Geometry: final body of the model. Coordinates: model frame, mm. A direction names the side the tool comes from. Coordinates: 2 decimals unless noted, no trailing zeros. Order: outer loops, then holes, each group sorted by start corner. A loop starts at its lowest first (then second) coordinate and runs counter-clockwise, first axis right, second up. Notation, with made-up numbers: (70.25, 65) -> (109.25, 65) arc R19 cw to (109.25, 89) -> close; hole circle Ø8 at (14.5, 6). An arc over 180 degrees is marked (long way). Use one line per item in the form item = value.
```python
from build123d import *

# Parameters (mm, degrees)
BOSS_EXTRUDE1_DEPTH = 14.5
CUT_EXTRUDE1_DEPTH  = 4
CUT_EXTRUDE2_DEPTH  = 4


with BuildPart() as part:
    # Sketch1 → Boss-Extrude1 (new body)
    with BuildSketch(Plane(origin=(0, 0, 0), x_dir=(0, 0, -1), z_dir=(1, 0, 0))):
        Polygon((0, 20), (0, 0), (20, 0), (20, 3), (3, 3), (3, 20), align=None)
    extrude(amount=-BOSS_EXTRUDE1_DEPTH)

    # Sketch2 → Cut-Extrude1 (cut, through all)
    with BuildSketch(Plane(origin=(0, 0, -3), x_dir=(-1, 0, 0), z_dir=(0, 0, -1))):
        with BuildLine():
            Line((5.5, 12.75), (9, 12.75))
            ThreePointArc((9, 12.75), (11.75, 10), (9, 7.25))
            Line((9, 7.25), (5.5, 7.25))
            ThreePointArc((5.5, 7.25), (2.75, 10), (5.5, 12.75))
        make_face()
    extrude(amount=-CUT_EXTRUDE1_DEPTH, mode=Mode.SUBTRACT)

    # Sketch3 → Cut-Extrude2 (cut, through all)
    with BuildSketch(Plane(origin=(0, 3, 0), x_dir=(1, 0, 0), z_dir=(0, 1, 0))):
        with BuildLine():
            Line((-5.5, 12.25), (-9, 12.25))
            ThreePointArc((-9, 12.25), (-11.75, 15), (-9, 17.75))
            Line((-9, 17.75), (-5.5, 17.75))
            ThreePointArc((-5.5, 17.75), (-2.75, 15), (-5.5, 12.25))
        make_face()
    extrude(amount=-CUT_EXTRUDE2_DEPTH, mode=Mode.SUBTRACT)


solid = part.part
```
1) Material intervals for probe 1 along Z at (x, y) = (-8.25, 14.75); probe 2 along Y at (x, z) = (-5.25, -4); probe 3 along Y at (x, z) = (-11, -2), sorted ascending. Write a range as from..to.
Results found:
probe_1 = -3..0
probe_2 = 0..3
probe_3 = 0..8.11, 11.89..20
2) Access query for faces 1 (the flat face through (-7, 3, -12)), 2 (the flat face through (-7, 7.25, -2)), 3 (the cylindrical face through (-11.75, 1.52, -14.94)). Directions: +Z, -Z, +X, -X, +Y, -Y. A direction counts if a zero-diameter tool reaches every point of the face in a straight line with its end or side. Return the directions, or none.
Results found:
face_1 = -Z, +X, -X, +Y
face_2 = +Z, -Z
face_3 = +Y, -Y
3) Section C-C, the plane y = 10. Output: boundary loops of the cut face in (x, z), and give its area (3 significant figures).
Results found:
outline = (-14.5, -3) -> (-11.75, -3) -> (-11.75, 0) -> (-14.5, 0) -> close; (-2.75, -3) -> (0, -3) -> (0, 0) -> (-2.75, 0) -> close
area = 16.5 mm2
4) Section B-B, the plane z = -15. Output: boundary loops of the cut face in (x, y).
Results found:
outline = (-14.5, 0) -> (-11.75, 0) -> (-11.75, 3) -> (-14.5, 3) -> close; (-2.75, 0) -> (0, 0) -> (0, 3) -> (-2.75, 3) -> close
5) Section D-D, the plane x = -2. Output: boundary loops of the cut face in (y, z).
Results found:
outline = (0, -20) -> (3, -20) -> (3, -3) -> (20, -3) -> (20, 0) -> (0, 0) -> close
6) Section A-A, the plane x = -7. Output: boundary loops of the cut face in (y, z).
Results found:
outline = (0, -20) -> (3, -20) -> (3, -17.75) -> (0, -17.75) -> close; (0, -12.25) -> (3, -12.25) -> (3, -3) -> (7.25, -3) -> (7.25, 0) -> (0, 0) -> close; (12.75, -3) -> (20, -3) -> (20, 0) -> (12.75, 0) -> close
7) Contact query for flat-ended pins moving along their axis: P1, Ø1, axis at x = -6.5, y = 4, coming from the +Z side; P2, Ø5, axis at x = -3, z = -11, coming from the +Y side. Output: stop coordinate, or through.
Results found:
P1 = 0
P2 = 3
8) Pull-direction query (Z, two-part tool) for faces 4 (the flat face through (-7, 2, -17.75)), 5 (the flat face through (-14.5, 6.3, -2.5)), 6 (the flat face through (-7, 13, -3)), 7 (the flat face through (-7, 2, -12.25)); classes: released by +Z, released by -Z, zero draft, split by the parting line, or undercut.
Results found:
face_4 = undercut
face_5 = zero draft
face_6 = released by -Z
face_7 = undercut
